Check sheet for the drawn part. Datum: minimum x, y, z corner. Units: mm. A direction names the side the tool comes from. Round coordinates to 2 decimals unless told otherwise and drop trailing zeros. Order: outer loops, then holes, each group sorted by start corner. A loop starts at its lowest first (then second) coordinate and runs counter-clockwise, first axis right, second up. Notation, with made-up numbers: (4, -39) - (23, -39) arc R15 ccw to (23, -24) - close; hole circle Ø8 at (5, -32.5). An arc over 180 degrees is marked (long way). Write each question's results on one line, items separated by ' | '.
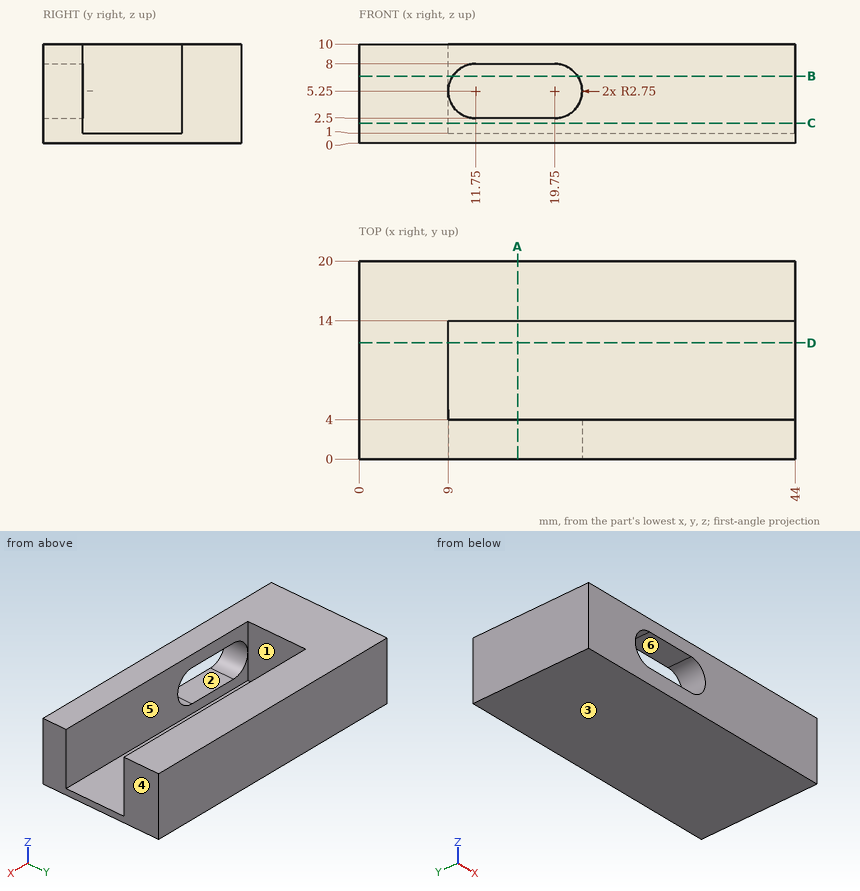
(1) Section check D-D (y = 11.75). Record the cut outline in (x, z).
Answers follow:
outline: (0, 0) - (44, 0) - (44, 1) - (9, 1) - (9, 10) - (0, 10) - close
(2) Draft check along X on the marked faces 4, 5 and 6. Enter one of: released by +X, released by -X, zero draft, split by the parting line, or undercut.
Answers follow:
face 4: released by +X | face 5: zero draft | face 6: undercut
(3) Section check B-B (z = 6.75). Record the cut outline in (x, y).
Answers follow:
outline: (0, 0) - (9.45, 0) - (9.45, 4) - (9, 4) - (9, 14) - (44, 14) - (44, 20) - (0, 20) - close; (22.05, 0) - (44, 0) - (44, 4) - (22.05, 4) - close
(4) Section check A-A (x = 16). Record the cut outline in (y, z), then the cut area to 3 significant figures.
Answers follow:
outline: (0, 0) - (20, 0) - (20, 10) - (14, 10) - (14, 1) - (4, 1) - (4, 2.5) - (0, 2.5) - close; (0, 8) - (4, 8) - (4, 10) - (0, 10) - close | area: 88.0 mm²
(5) Material ranges on line 1 (Y direction, x = 30, z = 4.25); line 2 (Z direction, x = 17, y = 2.25); line 3 (Z direction, x = 31, y = 10), recorded low to high.
Answers follow:
line 1: 0 to 4, 14 to 20 | line 2: 0 to 2.5, 8 to 10 | line 3: 0 to 1
(6) Access from +Z, -Z, +X, -X, +Y, -Y to the whole of each face (thin tool, end or side, straight path). Record for the marked faces 1, 2 and 3.
Answers follow:
face 1: +Z, +X | face 2: -Y | face 3: -Z, +X, -X, +Y, -Y
(7) Depth check by flat-ended pin: pin 1 Ø8 at (x, y) = (23, 9) entering from +Z. Enter the tip coordinate at first touch or a pass-through.
Answers follow:
pin 1: z = 1
(8) Section check C-C (z = 2). Record the cut outline in (x, y), then the cut area to 3 significant figures.
Answers follow:
outline: (0, 0) - (44, 0) - (44, 4) - (9, 4) - (9, 14) - (44, 14) - (44, 20) - (0, 20) - close | area: 530 mm²
